Geometry: final body of the model. Coordinates: model frame, mm. Face numbers are marked on the shaded views. A direction names the side the tool comes from. Give positions to 0.01 mm unless a question says otherwise; leave off trailing zeros. Write each loop counter-clockwise with the first axis right and the second up, starting at its lowest first coordinate (ties: lowest second). Pieces come first, ordered by that corner, then holes.
```python
from build123d import *

# Parameters (mm, degrees)
SKETCH2_W           = 6.4
SKETCH2_H           = 4.2
BOSS_EXTRUDE1_DEPTH = 1.5
SKETCH3_W           = 1.7
SKETCH3_H           = 4.2
BOSS_EXTRUDE2_DEPTH = 3.9
SKETCH4_W           = 0.15
SKETCH4_H           = 0.4
BOSS_EXTRUDE3_DEPTH = 3.7
BOSS_EXTRUDE4_DEPTH = 0.8
FILLET1_R           = 0.2
FILLET2_R           = 0.1
SKETCH6_W           = 0.45
SKETCH6_H           = 2.26
CUT_EXTRUDE1_DEPTH  = 0.3
SKETCH7_W           = 0.8
SKETCH7_H           = 3
CUT_EXTRUDE2_DEPTH  = 0.5
CHAMFER3_SIZE       = 0.7


with BuildPart() as part:
    # Sketch2 → Boss-Extrude1 (new body)
    with BuildSketch(Plane(origin=(0, 0, 0), x_dir=(1, 0, 0), z_dir=(0, 1, 0))):
        Rectangle(SKETCH2_W, SKETCH2_H)
    extrude(amount=BOSS_EXTRUDE1_DEPTH)

    # Sketch3 → Boss-Extrude2 (add)
    with BuildSketch(Plane(origin=(0, 1.5, 0), x_dir=(1, 0, 0), z_dir=(0, 1, 0))):
        with Locations((-2.35, 0)):
            Rectangle(SKETCH3_W, SKETCH3_H)
        with Locations((2.35, 0)):
            Rectangle(SKETCH3_W, SKETCH3_H)
    extrude(amount=BOSS_EXTRUDE2_DEPTH)

    # Sketch4 → Boss-Extrude3 (add)
    with BuildSketch(Plane.XZ):
        with Locations((2.5, 1.27)):
            Rectangle(SKETCH4_W, SKETCH4_H)
        with Locations((-2.5, 1.27)):
            Rectangle(SKETCH4_W, SKETCH4_H)
        with Locations((2.5, -1.27)):
            Rectangle(SKETCH4_W, SKETCH4_H)
        with Locations((-2.5, -1.27)):
            Rectangle(SKETCH4_W, SKETCH4_H)
    extrude(amount=BOSS_EXTRUDE3_DEPTH)

    # Sketch5 → Boss-Extrude4 (add)
    with BuildSketch(Plane.XZ):
        with BuildLine():
            Line((-0.606217783, 1.6), (0.606217783, 1.6))
            ThreePointArc((0.606217783, 1.6), (0, 0.55), (-0.606217783, 1.6))
        make_face()
        with BuildLine():
            Line((-0.357071421, -1.6), (0.357071421, -1.6))
            ThreePointArc((0.357071421, -1.6), (0, -0.75), (-0.357071421, -1.6))
        make_face()
    extrude(amount=BOSS_EXTRUDE4_DEPTH)

    # Fillet1
    fillet1_edges = [part.edges().sort_by_distance(p)[0] for p in [
        (0, -0.8, 0.55),
        (0, -0.8, 1.6),
    ]]
    fillet(fillet1_edges, radius=FILLET1_R)

    # Fillet2
    fillet2_edges = [part.edges().sort_by_distance(p)[0] for p in [
        (0, -0.8, -0.75),
        (0, -0.8, -1.6),
    ]]
    fillet(fillet2_edges, radius=FILLET2_R)

    # Sketch6 → Cut-Extrude1 (cut)
    with BuildSketch(Plane(origin=(-1.5, 0, 0), x_dir=(0, 0, -1), z_dir=(1, 0, 0))):
        with Locations((0, 4.27)):
            Rectangle(SKETCH6_W, SKETCH6_H)
    cut_extrude1 = extrude(amount=-CUT_EXTRUDE1_DEPTH, mode=Mode.SUBTRACT)

    # Sketch7 → Cut-Extrude2 (cut)
    with BuildSketch(Plane.ZY.offset(3.2)):
        with Locations((0, 3.9)):
            Rectangle(SKETCH7_W, SKETCH7_H)
    cut_extrude2 = extrude(amount=-CUT_EXTRUDE2_DEPTH, mode=Mode.SUBTRACT)

    # Chamfer3
    chamfer3_edges = [part.edges().sort_by_distance(p)[0] for p in [
        (2.35, 5.4, -2.1),
        (-2.35, 5.4, -2.1),
    ]]
    chamfer(chamfer3_edges, length=CHAMFER3_SIZE)

    # Mirror5: Cut-Extrude1, Cut-Extrude2 across plane
    add(cut_extrude1.mirror(Plane(origin=(0, 0, 0), x_dir=(0, 0, 1), z_dir=(1, 0, 0))), mode=Mode.SUBTRACT)
    add(cut_extrude2.mirror(Plane(origin=(0, 0, 0), x_dir=(0, 0, 1), z_dir=(1, 0, 0))), mode=Mode.SUBTRACT)


solid = part.part
```
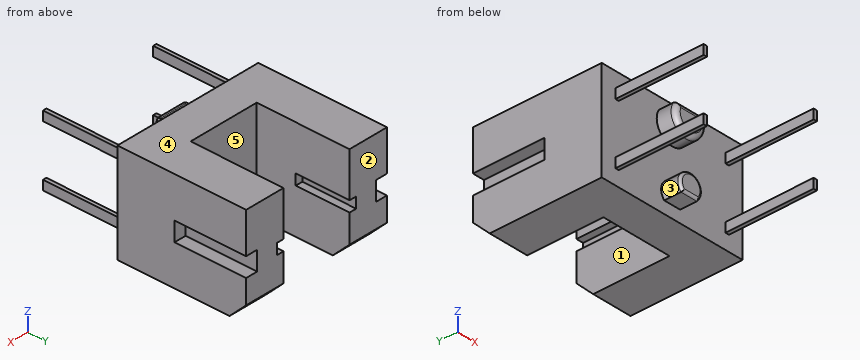
Item 1: Reachability of the marked faces 1 and 2 from +Z, -Z, +X, -X, +Y, -Y: full face, straight path, thin tool, end or side. Return the list, or none.
Found:
face 1: +Z, -Z, +Y
face 2: +Z, -Z, +X, -X, +Y
Item 2: Section C-C, the plane x = 0. Return the cut outline in (y, z), plus the area to 3 significant figures.
Found:
outline: (-0.8, -1.5) arc R0.1 ccw to (-0.7, -1.6) - (0, -1.6) - (0, -2.1) - (1.5, -2.1) - (1.5, 2.1) - (0, 2.1) - (0, 1.6) - (-0.6, 1.6) arc R0.2 ccw to (-0.8, 1.4) - (-0.8, 0.75) arc R0.2 ccw to (-0.6, 0.55) - (0, 0.55) - (0, -0.75) - (-0.7, -0.75) arc R0.1 ccw to (-0.8, -0.85) - close
area: 7.80 mm2
Item 3: Pull-direction query (Z, two-part tool) for the marked faces 3, 4 and 5; classes: +Z half, -Z half, draft (parallel to the pull), parting line (faces both ways), or undercut.
Found:
face 3: undercut
face 4: +Z half
face 5: draft
Item 4: Section A-A, the plane y = -0.25. Return the cut outline in (x, z) (3 decimals).
Found:
outline: (-2.575, -1.47) - (-2.425, -1.47) - (-2.425, -1.07) - (-2.575, -1.07) - close; (-2.575, 1.07) - (-2.425, 1.07) - (-2.425, 1.47) - (-2.575, 1.47) - close; (-0.606, 1.6) arc R0.7 ccw (long way) to (0.606, 1.6) - close; (-0.357, -1.6) - (0.357, -1.6) arc R0.5 ccw (long way) to start; (2.425, -1.47) - (2.575, -1.47) - (2.575, -1.07) - (2.425, -1.07) - close; (2.425, 1.07) - (2.575, 1.07) - (2.575, 1.47) - (2.425, 1.47) - close
Item 5: Line query: L1, parallel to X at y = 3.5, z = -1.2; L2, parallel to Y at x = 1.25, z = -1.65; L3, parallel to Y at x = 2, z = -1. Output: solid intervals per line, ascending.
Found:
L1: x = -3.2 to -1.5, 1.5 to 3.2
L2: y = 0 to 1.5
L3: y = 0 to 5.4
Item 6: Section D-D, the plane y = -1.5. Return the cut outline in (x, z) (3 decimals), plus the area to 3 significant figures.
Found:
outline: (-2.575, -1.47) - (-2.425, -1.47) - (-2.425, -1.07) - (-2.575, -1.07) - close; (-2.575, 1.07) - (-2.425, 1.07) - (-2.425, 1.47) - (-2.575, 1.47) - close; (2.425, -1.47) - (2.575, -1.47) - (2.575, -1.07) - (2.425, -1.07) - close; (2.425, 1.07) - (2.575, 1.07) - (2.575, 1.47) - (2.425, 1.47) - close
area: 0.240 mm2
Item 7: Pin query (flat end, axial travel): pin 1 Ø1 at (x, z) = (-1, 1) entering from -Y; pin 2 Ø0.5 at (y, z) = (4.5, 0) entering from +X; pin 3 Ø1.5 at (x, z) = (0, 1) entering from +Y. Return the tip coordinate at first contact, or that it passes through.
Found:
pin 1: stops at y = -0.8
pin 2: stops at x = 2.7
pin 3: stops at y = 1.5
Item 8: Section B-B, the plane z = 0.05. Return the cut outline in (x, y).
Found:
outline: (-3.2, 0) - (3.2, 0) - (3.2, 2.4) - (2.7, 2.4) - (2.7, 5.4) - (1.8, 5.4) - (1.8, 3.14) - (1.5, 3.14) - (1.5, 1.5) - (-1.5, 1.5) - (-1.5, 3.14) - (-1.8, 3.14) - (-1.8, 5.4) - (-2.7, 5.4) - (-2.7, 2.4) - (-3.2, 2.4) - close
